```python
from build123d import *

# Parameters (mm, degrees)
SKETCH2_R           = 3.175
BOSS_EXTRUDE1_DEPTH = 20.32
SKETCH3_R           = 4.445
BOSS_EXTRUDE2_DEPTH = 3.175
SKETCH4_R           = 3.175
CUT_EXTRUDE1_DEPTH  = 6.35


with BuildPart() as part:
    # Sketch2 → Boss-Extrude1 (new body)
    with BuildSketch(Plane.XY):
        Circle(SKETCH2_R)
    extrude(amount=-BOSS_EXTRUDE1_DEPTH)

    # Sketch3 → Boss-Extrude2 (add, symmetric)
    with BuildSketch(Plane(origin=(0, 0, 0), x_dir=(0, 0, -1), z_dir=(1, 0, 0))):
        Circle(SKETCH3_R)
    extrude(amount=BOSS_EXTRUDE2_DEPTH, both=True)

    # Sketch4 → Cut-Extrude1 (cut)
    with BuildSketch(Plane(origin=(3.175, 0, 0), x_dir=(0, 0, -1), z_dir=(1, 0, 0))):
        Circle(SKETCH4_R)
    extrude(amount=-CUT_EXTRUDE1_DEPTH, mode=Mode.SUBTRACT)


solid = part.part
```
The listing builds one solid part. Answer for the finished solid, in the listing's coordinates (mm). A direction names the side the tool comes from. Round coordinates to 2 decimals unless told otherwise and drop trailing zeros. Loops run counter-clockwise (first coordinate to the right, second up) from the corner with the lowest first, then second, coordinate; pieces in that order, holes last.
1) For a pull along Y with two mould halves and no side action, classify faces 1 (the face through (0.04, -3.1, 0.69)), 2 (the face through (3.175, -3, -2)), 3 (the face through (0.04, 0.2, 4.44)) as released by +Y, released by -Y, zero draft, split by the parting line, or undercut.
Outcome:
face 1: undercut
face 2: zero draft
face 3: split by the parting line
2) Given P1, Ø1, axis at y = -3, z = -8.5, coming from the +X side; P2, Ø5, axis at y = 2, z = -6.5, coming from the +X side (3 decimals); P3, Ø3, axis at x = -1, z = -6, coming from the +Y side (3 decimals); P4, Ø4, axis at y = 0, z = 0, coming from the +X side, each flat-ended and moving along its own axis, determine where each tip first touches the part or whether it passes through.
Outcome:
P1: stops at x = 1.96
P2: stops at x = 3.175
P3: stops at y = 3.175
P4: passes through
3) A cutting plane is placed at A-A on z = 0. Determine the outline of the cut face in (x, y) (3 decimals), plus the area to 3 significant figures.
Outcome:
outline: (-3.175, -4.445) - (3.175, -4.445) - (3.175, -3.175) - (-3.175, -3.175) - close; (-3.175, 3.175) - (3.175, 3.175) - (3.175, 4.445) - (-3.175, 4.445) - close
area: 16.1 mm2
4) Consider line 1 (Y direction, x = 0, z = 0) (3 decimals); line 2 (Y direction, x = -1, z = 1.25); line 3 (Z direction, x = 1.5, y = -2.25). Determine where each line is inside the solid, lowest interval first.
Outcome:
line 1: y = -4.445 to -3.175, 3.175 to 4.445
line 2: y = -4.27 to -2.92, 2.92 to 4.27
line 3: z = -20.32 to -2.24, 2.24 to 3.83
5) A cutting plane is placed at B-B on y = -1.75. Determine the outline of the cut face in (x, z) (3 decimals).
Outcome:
outline: (-3.175, -4.086) - (-2.649, -4.086) - (-2.649, -20.32) - (2.649, -20.32) - (2.649, -4.086) - (3.175, -4.086) - (3.175, -2.649) - (-3.175, -2.649) - close; (-3.175, 2.649) - (3.175, 2.649) - (3.175, 4.086) - (-3.175, 4.086) - close
6) A cutting plane is placed at C-C on x = -2.5. Determine the outline of the cut face in (y, z) (3 decimals), plus the area to 3 significant figures.
Outcome:
outline: (-1.957, -20.32) - (1.957, -20.32) - (1.957, -3.991) arc R4.445 ccw (long way) to (-1.957, -3.991) - close; hole circle Ø6.35 at (0, 0)
area: 93.1 mm2
7) A cutting plane is placed at D-D on z = -9. Determine the outline of the cut face in (x, y) (3 decimals), plus the area to 3 significant figures.
Outcome:
outline: circle Ø6.35 at (0, 0)
area: 31.7 mm2
8) For faces 4 (the face through (0, 0, -20.32)), 5 (the face through (-0.41, 3.15, -11.59)), determine the directions among +Z, -Z, +X, -X, +Y, -Y from which every point of the face is accessible in a straight line to the end or side of a thin tool.
Outcome:
face 4: -Z, +X, -X, +Y, -Y
face 5: -Z
